The listing builds one solid part. Answer for the finished solid, in the listing's coordinates (mm). A direction names the side the tool comes from. Coordinates: 2 decimals unless noted, no trailing zeros. Order: outer loops, then holes, each group sorted by start corner. A loop starts at its lowest first (then second) coordinate and runs counter-clockwise, first axis right, second up. Notation, with made-up numbers: (-15.75, 84.5) -> (29.25, 84.5) arc R7 ccw to (29.25, 88.5) -> close; hole circle Ø3 at (79.5, -6.5). An arc over 180 degrees is marked (long way). Return JSON: item names as keys, results as strings.
Autodesk Fusion 360 part; units mm, degrees
sketch "スケッチ1" plane through (0, 0, 0) normal (0, 0, 1) x (1, 0, 0)
  line L0 (0, 0) -> (-45, 0)
  line L1 (-45, 0) -> (-45, -110)
  line L2 (-45, -110) -> (0, -110)
  line L3 (0, -110) -> (0, 0)
  circle A0 centre (-35, -25) radius 4.5
  circle A1 centre (-10, -25) radius 4.5
  dimension "d1" = 45
  dimension "d2" = 110
  dimension "d3" = 9
  dimension "d4" = 9
  dimension "d5" = 25
  dimension "d6" = 10
  dimension "d7" = 25
extrude "押し出し1" add sketch "スケッチ1" against normal blind 15 contours L0 L1 L2 L3 | A0 | A1
extrude "押し出し2" cut sketch "スケッチ1" against normal blind 15 contours A0 | A1
sketch "スケッチ2" plane through (0, 0, 0) normal (0, 0, 1) x (1, 0, 0)
  line L0 (0, -95) -> (-45, -95)
  line L1 (-45, -95) -> (-45, -110)
  line L2 (-45, -110) -> (0, -110)
  line L3 (0, -110) -> (0, -95)
  line L4 (0, -110) -> (0, 0)
  point P0 (-45, -110)
  dimension "d12" = 15
extrude "押し出し3" add sketch "スケッチ2" along normal blind 105
sketch "スケッチ3" plane through (0, 0, 0) normal (1, 0, 0) x (0, 1, 0)
  line L0 (-110, 105) -> (-110, -15)
  line L1 (-110, -15) -> (0, -15)
  line L2 (0, -15) -> (0, 0)
  line L3 (0, 0) -> (-95, 0)
  line L4 (-95, 0) -> (-95, 105)
  line L5 (-95, 105) -> (-110, 105)
  line L6 (-110, 95) -> (-102, 95)
  line L7 (-102, 95) -> (-110, 103)
  line L8 (-102, 95) -> (-110, 87)
  circle A0 centre (-117.5091, 95.717) radius 11
  line L9 (-146.8307, 84.717) -> (-108.4644, 84.717)
  line L10 (-108.4644, 84.717) -> (-108.4644, 71.717)
  line L11 (-108.4644, 71.717) -> (-146.8307, 71.717)
  line L12 (-146.8307, 71.717) -> (-146.8307, 84.717)
  circle A1 centre (-117.5091, 60.717) radius 11
  line L13 (-110, 60) -> (-102, 60)
  line L14 (-102, 60) -> (-110, 68)
  line L15 (-102, 60) -> (-110, 52)
  circle A2 centre (-117.5091, 60.717) radius 13
  circle A3 centre (-117.5091, 36.717) radius 11
  line L16 (-102, 36) -> (-110, 28)
  line L17 (-102, 36) -> (-110, 44)
  line L18 (-102, 1) -> (-110, 9)
  line L19 (-102, 1) -> (-110, -7)
  circle A4 centre (-117.5091, 1.717) radius 13
  circle A5 centre (-113.2021, 95.093) radius 7.5
  circle A6 centre (-113.2568, 60.0071) radius 7.5
  dimension "d15" = 8
  dimension "d16" = 45
  dimension "d17" = 22
  dimension "d18" = 13
  dimension "d19" = 38.3662
  dimension "d20" = 22
  dimension "d21" = 8
  dimension "d22" = 45
  dimension "d23" = 35
  dimension "d24" = 26
  dimension "d27" = 0
  dimension "d28" = -59
  dimension "d29" = 2
  dimension "d32" = 15
  dimension "d33" = 15
extrude "押し出し4" cut sketch "スケッチ3" against normal blind 50 contours L0 L18 L19 A4 | L18 L19 A4 | L0 A3 L16 L17 | L0 A3 L17 | L0 A1 L13 L15 A2 A6 | L13 L15 A2 | L0 A1 A6 | L13 L14 A2 | A1 L13 L14 A2 A6 | L0 A1 L14 A6 | L0 A1 L13 A6 | A1 L13 A6 | A1 L13 A6 | L0 A1 L13 A6 | L0 L6 L8 A0 A5 | L0 A0 A5 | L0 L7 A0 A5 | L6 L7 A0 A5 | L0 L6 A0 A5 | L6 A0 A5 | L0 L6 A0 A5 | L6 A0 A5 picked at (-109.6585, 34.1515) picked at (-109.8639, 53.0034) picked at (-109.8537, 88.034)
sketch "スケッチ4" plane through (0, -110, 0) normal (0, -1, 0) x (1, 0, 0)
  line L0 (-45, 68) -> (0, 68)
  line L1 (0, 68) -> (0, 87)
  line L2 (0, 87) -> (-45, 87)
  line L3 (-45, 87) -> (-45, 68)
  circle A0 centre (-35, 77.5) radius 4
  circle A1 centre (-10, 77.5) radius 4
  line L4 (-22.5, 77.5) -> (-22.5, 71.9777)
  line L5 (-45, 105) -> (0, 105)
  circle A2 centre (-35, 18.5) radius 4
  circle A3 centre (-10, 18.5) radius 4
  dimension "d34" = 8
  dimension "d35" = 8
  dimension "d36" = 25
  dimension "d37" = 12.5
  dimension "d38" = 45
  dimension "d39" = 27.5
  dimension "d42" = 0
  dimension "d43" = -59
extrude "押し出し5" cut sketch "スケッチ4" against normal blind 15 contours A0 | A1 | A2 | A3
equation "d13 = 120 mm - 15 mm"
equation "d37 = ( 25 / 2 ) * 1 mm"
Item 1: The part is cut by section A-A on z = 77.5. Determine the outline of the cut face in (x, y).
Answer list:
{"outline": "(-45, -110) -> (-39, -110) -> (-39, -95) -> (-45, -95) -> close; (-31, -110) -> (-14, -110) -> (-14, -95) -> (-31, -95) -> close; (-6, -110) -> (0, -110) -> (0, -95) -> (-6, -95) -> close"}
Item 2: The part is cut by section D-D on y = -100.5. Determine the outline of the cut face in (x, z), plus the area to 3 significant figures.
Answer list:
{"outline": "(-45, -15) -> (0, -15) -> (0, 105) -> (-45, 105) -> close; hole circle Ø8 at (-35, 18.5); hole circle Ø8 at (-35, 77.5); hole circle Ø8 at (-10, 18.5); hole circle Ø8 at (-10, 77.5)", "area": "5,200 mm2"}
Item 3: The part is cut by section C-C on x = -35. Count the separate pieces of the cut face and the enclosed holes in it, plus the area to 3 significant figures.
Answer list:
{"separate pieces": "4", "enclosed holes": "0", "area": "2,590 mm2"}
Item 4: Flat-ended cylindrical pins translate along their axes: pin 1 (11.5 mm diameter, centred on x = -35, y = -25, fed in from +Z); pin 2 (22.5 mm diameter, centred on x = -12.5, z = 44, fed in from +Y); pin 3 (2 mm diameter, centred on x = -13, z = 30.5, fed in from -Y). Find the tip coordinate at first contact, or state that the pin passes through.
Answer list:
{"pin 1": "z = 0", "pin 2": "y = -95", "pin 3": "y = -108.5"}
Item 5: Find the intervals of material crossed by probe 1 along Z at (x, y) = (-35, -98.25); probe 2 along Z at (x, y) = (-7, -97); probe 3 along Z at (x, y) = (-20.5, -72), in increasing order.
Answer list:
{"probe 1": "-15 to 14.5, 22.5 to 73.5, 81.5 to 105", "probe 2": "-15 to 15.85, 21.15 to 74.85, 80.15 to 105", "probe 3": "-15 to 0"}
Item 6: The part is cut by section B-B on y = -25. Determine the outline of the cut face in (x, z).
Answer list:
{"outline": "(-45, -15) -> (-39.5, -15) -> (-39.5, 0) -> (-45, 0) -> close; (-30.5, -15) -> (-14.5, -15) -> (-14.5, 0) -> (-30.5, 0) -> close; (-5.5, -15) -> (0, -15) -> (0, 0) -> (-5.5, 0) -> close"}
Item 7: Determine the mould class of faces 1 (the flat face through (-23, -110, 48)), 2 (the flat face through (0, -96, 27)), 3 (the cylindrical face through (-10.521, -102.605, 22.466)) for opening direction X: pulls with the +X half, pulls with the -X half, needs draft (parallel to the pull), parting line crosses it, or undercut.
Answer list:
{"face 1": "needs draft", "face 2": "pulls with the +X half", "face 3": "undercut"}
Item 8: Which of the six approach directions +Z, -Z, +X, -X, +Y, -Y give full straight-line access (tool end or side, diameter ignored) to faces 4 (the flat face through (-22, 0, -7)), 5 (the flat face through (-22, -106, 99)), 6 (the flat face through (-23, -47, 0))?
Answer list:
{"face 4": "+Z, -Z, +X, -X, +Y", "face 5": "+X, -X, -Y", "face 6": "+Z, +X, -X, +Y"}
